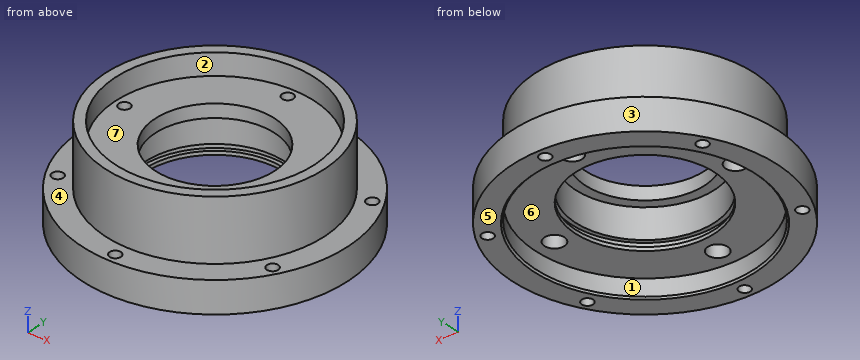
```python
from build123d import *

# Parameters (mm, degrees)
SKETCH_2_W               = 4
SKETCH_2_H               = 1.7
SKETCH_6_R               = 1.7
CUT_EXTRUDE_1_DEPTH      = 64.118935352
PATTERN_CIRCULAR_1_COUNT = 6
CHAMFER_1_SIZE           = 0.5
PATTERN_CIRCULAR_2_COUNT = 4


with BuildPart() as part:
    # Sketch 1 → Revolve 1 (revolve)
    with BuildSketch(Plane(origin=(0, 0, 0), x_dir=(0, 0, -1), z_dir=(1, 0, 0)), mode=Mode.PRIVATE) as revolve_1_sk:
        Polygon((0, 30), (0, 18), (4, 18), (4, 21), (13, 21), (13, 22.25), (14.9, 22.25), (14.9, 21), (16, 21), (16, 33), (21.5, 33), (21.5, 40), (12, 40), (12, 33), (-6.5, 33), (-6.5, 30), align=None)
    revolve(revolve_1_sk.sketch.rotate(Axis((0, 0, 0), (0, 0, -1)), 90), axis=Axis((0, 0, 0), (0, 0, -1)))

    # Sketch 2 → Cut-Revolve 2 (revolve, cut)
    with BuildSketch(Plane(origin=(0, 0, 0), x_dir=(0, 0, -1), z_dir=(1, 0, 0)), mode=Mode.PRIVATE) as cut_revolve_2_sk:
        Polygon((4, 28.7), (4, 27), (16, 27), (16, 30), (4, 30), align=None)
        with Locations((2, 27.85)):
            Rectangle(SKETCH_2_W, SKETCH_2_H)
    cut_revolve_2 = revolve(cut_revolve_2_sk.sketch.rotate(Axis((0, 27, 0), (0, 0, -1)), 90), axis=Axis((0, 27, 0), (0, 0, -1)), mode=Mode.SUBTRACT)

    # Sketch 6 → Cut-Extrude 1 (cut, symmetric)
    with BuildSketch(Plane(origin=(0, 0, -21.5), x_dir=(-1, 0, 0), z_dir=(0, 0, -1))):
        with Locations((0, 37)):
            Circle(SKETCH_6_R)
    cut_extrude_1 = extrude(amount=CUT_EXTRUDE_1_DEPTH, both=True, mode=Mode.SUBTRACT)

    # Pattern Circular 1: Cut-Extrude 1 ×6 about axis
    pattern_circular_1_axis = Axis((0, 0, 0), (0, 0, 1))
    for i in range(1, PATTERN_CIRCULAR_1_COUNT):
        add(cut_extrude_1.rotate(pattern_circular_1_axis, i * 360 / PATTERN_CIRCULAR_1_COUNT), mode=Mode.SUBTRACT)

    # Chamfer 1
    chamfer_1_edges = [part.edges().sort_by_distance(p)[0] for p in [
        (-33, 0, -21.5),
    ]]
    chamfer(chamfer_1_edges, length=CHAMFER_1_SIZE)

    # Pattern Circular 2: Cut-Revolve 2 ×4 about axis
    pattern_circular_2_axis = Axis((0, 0, 0), (0, 0, 1))
    for i in range(1, PATTERN_CIRCULAR_2_COUNT):
        add(cut_revolve_2.rotate(pattern_circular_2_axis, i * 360 / PATTERN_CIRCULAR_2_COUNT), mode=Mode.SUBTRACT)


solid = part.part
```
Verification items for the finished model (mm, model axes). Face numbers are marked on the shaded views. A direction names the side the tool comes from. Coordinates: 2 decimals unless noted, no trailing zeros. Write each loop counter-clockwise with the first axis right and the second up, starting at its lowest first coordinate (ties: lowest second). Pieces come first, ordered by that corner, then holes. Notation, with made-up numbers: (-9, -28.75) - (36, -28.75) arc R16 cw to (36, -8.75) - close; hole circle Ø7 at (-30.75, -8). An arc over 180 degrees is marked (long way). One line per question, with ' | ' between items. Start each with the question number.
1. Material ranges on line 1 along Y through (x, z) = (0, -9.75); line 2 along Y through (x, z) = (0, -0.75); line 3 along Y through (x, z) = (0, 5.25), recorded low to high.
2. Access from +Z, -Z, +X, -X, +Y, -Y to the whole of each face (thin tool, end or side, straight path). Record for the marked faces 5, 6 and 7.
3. Section check A-A (z = -8.75). Enter the section's corners in (x, y), plus the area to 3 significant figures.
4. Section check C-C (z = -18.5). Enter the section's corners in (x, y), plus the area to 3 significant figures.
5. Section check D-D (z = 4). Enter the section's corners in (x, y), plus the area to 3 significant figures.
6. Draft check along X on the marked faces 1, 2, 3 and 4. Enter one of: released by +X, released by -X, zero draft, split by the parting line, or undercut.
7. Section check B-B (y = -37). Enter the section's corners in (x, z).
8. Gauge pin test, flat ends, axial feed: P1, Ø8, axis at y = -22, z = -12.5, coming from the -X side; P2, Ø3, axis at x = -32.04, y = 18.5, coming from the -Z side; P3, Ø8, axis at x = 4, y = 23, coming from the -Z side; P4, Ø4.5, axis at x = 27, y = 0, coming from the +Z side. Record the tip position at first contact, or that the pin passes through.
Computed values:
1) line 1: -33 to -30, -24 to -21, 21 to 24, 30 to 33 | line 2: -33 to -28.7, -25.3 to -18, 18 to 25.3, 28.7 to 33 | line 3: -33 to -30, 30 to 33
2) face 5: -Z, +X, -X, +Y, -Y | face 6: -Z | face 7: +Z
3) outline: circle Ø66 at (0, 0); hole circle Ø6 at (-27, 0); hole circle Ø42 at (0, 0); hole circle Ø6 at (0, -27); hole circle Ø6 at (0, 27); hole circle Ø6 at (27, 0) | area: 1,920 mm²
4) outline: circle Ø80 at (0, 0); hole circle Ø3.4 at (-32.04, -18.5); hole circle Ø3.4 at (-32.04, 18.5); hole circle Ø66 at (0, 0); hole circle Ø3.4 at (0, -37); hole circle Ø3.4 at (0, 37); hole circle Ø3.4 at (32.04, -18.5); hole circle Ø3.4 at (32.04, 18.5) | area: 1,550 mm²
5) outline: circle Ø66 at (0, 0); hole circle Ø60 at (0, 0) | area: 594 mm²
6) face 1: undercut | face 2: undercut | face 3: split by the parting line | face 4: zero draft
7) outline: (-15.2, -21.5) - (-1.7, -21.5) - (-1.7, -12) - (-15.2, -12) - close; (1.7, -21.5) - (15.2, -21.5) - (15.2, -12) - (1.7, -12) - close
8) P1: x = -35.72 | P2: through | P3: z = -16 | P4: z = 0
